from build123d import *

# Parameters (mm, degrees)
F0_W     = 23
F0_H     = 20
F1_DEPTH = 5
F2_R     = 2.025
F2_R_2   = 3.175
F3_DEPTH = 25
F5_D     = 5
F7_D     = 2.4
F7_DEPTH = 5
F7_TIP   = 0.7210327428
F9_D     = 2.4
F9_DEPTH = 5
F9_TIP   = 0.7210327428


with BuildPart() as f1:
    # F0 (on Top) → F1 (new body, symmetric)
    with BuildSketch(Plane.XY):
        Rectangle(F0_W, F0_H)
    extrude(amount=F1_DEPTH, both=True)

    # F2 (on face) → F3 (cut)
    with BuildSketch(Plane.XZ.offset(10)):
        with Locations((-7.075, 0)):
            Circle(F2_R)
        with Locations((5.925, 0)):
            Circle(F2_R_2)
    extrude(amount=-F3_DEPTH, mode=Mode.SUBTRACT)

    # F5 (through all)
    with Locations(Plane.XY.offset(5)):
        with Locations((-1.15, 0)):
            Hole(F5_D / 2)

    # F7
    with Locations(Plane(origin=(-11.5, 0, 0), x_dir=(0, -1, 0), z_dir=(-1, 0, 0))):
        with Locations((0, 0)):
            Hole(F7_D / 2, depth=F7_DEPTH)
            with Locations((0, 0, -(F7_DEPTH + F7_TIP / 2))):  # 118° drill point
                Cone(0, F7_D / 2, F7_TIP, mode=Mode.SUBTRACT)

    # F9
    with Locations(Plane.YZ.offset(11.5)):
        with Locations((0, 0)):
            Hole(F9_D / 2, depth=F9_DEPTH)
            with Locations((0, 0, -(F9_DEPTH + F9_TIP / 2))):  # 118° drill point
                Cone(0, F9_D / 2, F9_TIP, mode=Mode.SUBTRACT)


solid = f1.part
Work out the finished part from the listing and answer in its coordinate system (mm). A direction names the side the tool comes from. Round coordinates to 2 decimals unless told otherwise and drop trailing zeros. Write each loop counter-clockwise with the first axis right and the second up, starting at its lowest first coordinate (ties: lowest second). Pieces come first, ordered by that corner, then holes. Notation, with made-up numbers: M -7.75,64 L 20.25,64 A23 cw 20.25,92 Z; hole C -0.75,-26 d1. An arc over 180 degrees is marked long. Use a Markdown table: item, result.
1) The part is cut by section C-C on z = 2.75. Give the vertices of the cut face in (x, y).
Taken from the geometry:
| item | result |
|---|---|
| outline | M -11.5,-10 L 4.34,-10 L 4.34,10 L -11.5,10 Z; M 7.51,-10 L 11.5,-10 L 11.5,10 L 7.51,10 Z; hole C -1.15,0 d5 |
2) The part is cut by section B-B on x = -1.15. Give the vertices of the cut face in (y, z).
Taken from the geometry:
| item | result |
|---|---|
| outline | M -10,-5 L -2.5,-5 L -2.5,5 L -10,5 Z; M 2.5,-5 L 10,-5 L 10,5 L 2.5,5 Z |
3) Which of the six approach directions +Z, -Z, +X, -X, +Y, -Y give full straight-line access (tool end or side, diameter ignored) to faces 1 (the face through (0, -10, 0)), 2 (the face through (10.164, -1.145, 0.36))?
Taken from the geometry:
| item | result |
|---|---|
| face 1 | +Z, -Z, +X, -X, -Y |
| face 2 | +X |
4) The part is cut by section A-A on z = 0. Give the vertices of the cut face in (x, y).
Taken from the geometry:
| item | result |
|---|---|
| outline | M -11.5,-10 L -9.1,-10 L -9.1,-1.2 L -11.5,-1.2 Z; M -11.5,1.2 L -9.1,1.2 L -9.1,10 L -11.5,10 Z; M -5.05,-10 L 2.75,-10 L 2.75,10 L -5.05,10 Z; M 9.1,-10 L 11.5,-10 L 11.5,-1.2 L 9.1,-1.2 Z; M 9.1,1.2 L 11.5,1.2 L 11.5,10 L 9.1,10 Z; hole C -1.15,0 d5 |
5) Consider line 1 (Y direction, x = -1.15, z = -2); line 2 (Z direction, x = 9.95, y = 0); line 3 (X direction, y = -6.25, z = 1.5). Determine where each line is inside the solid, lowest interval first. Write a range as [from, to].
Taken from the geometry:
| item | result |
|---|---|
| line 1 | y = [-10, -2.5], [2.5, 10] |
| line 2 | z = [-5, -1.2], [1.2, 5] |
| line 3 | x = [-11.5, -8.44], [-5.71, 3.13], [8.72, 11.5] |
6) Determine the mould class of faces 3 (the face through (-10.084, 1.145, 0.36)), 4 (the face through (-11.5, 0, 2)), 5 (the face through (2, 0, 5)) for opening direction Z: pulls with the +Z half, pulls with the -Z half, needs draft (parallel to the pull), parting line crosses it, or undercut.
Taken from the geometry:
| item | result |
|---|---|
| face 3 | undercut |
| face 4 | needs draft |
| face 5 | pulls with the +Z half |
